```python
from build123d import *

# Parameters (mm, degrees)
F0_R          = 6.75
F0_R_2        = 2.15
F1_DEPTH      = 6
F1_DEPTH_BACK = 6
F3_START      = 5
F3_DEPTH      = 25
F4_SIZE2      = 3
F4_SIZE       = 1


with BuildPart() as f1:
    # F0 (on Top) → F1 (new body, two sides)
    with BuildSketch(Plane.XY) as f1_sk:
        Circle(F0_R)
        Circle(F0_R_2, mode=Mode.SUBTRACT)
    extrude(amount=F1_DEPTH)
    extrude(f1_sk.sketch, amount=-F1_DEPTH_BACK)

    # F2 (on Front) → F3 (join)
    with BuildSketch(Plane.XZ.offset(F3_START)):
        with BuildLine():
            ThreePointArc((1.5745130543, -4.2155555556), (3.6969790873, -2.5656082374), (4.5, 0))
            ThreePointArc((4.5, 0), (-2.5656082374, 3.6969790873), (-1.5745130543, -4.2155555556))
            ThreePointArc((-1.5745130543, -4.2155555556), (0, -2.9), (1.5745130543, -4.2155555556))
        make_face()
    extrude(amount=F3_DEPTH)

    # F4
    f4_edges = [f1.edges().sort_by_distance(p)[0] for p in [
        (0, -30, 4.5),
    ]]
    f4_side = f1.faces().sort_by_distance((0, -30, 0.234076))[0]
    chamfer(f4_edges, length=F4_SIZE, length2=F4_SIZE2, reference=f4_side)


solid = f1.part
```
Source: CAD feature listing. Evaluate the final solid. Frame: model axes, mm. A direction names the side the tool comes from. Give positions to 0.01 mm unless a question says otherwise; leave off trailing zeros. Loops run counter-clockwise (first coordinate to the right, second up) from the corner with the lowest first, then second, coordinate; pieces in that order, holes last. Notation, with made-up numbers: (-30.5, 65.25) - (-8.5, 65.25) arc R26 cw to (-8.5, 82.25) - close; hole circle Ø8 at (-21.5, -26). An arc over 180 degrees is marked (long way). Use CSV: the item, a comma, the result in double quotes. Start each with the question number.
1. Section C-C (y = -21.5). Output: boundary loops of the cut face in (x, z).
2. Reachability of faces 1 (the flat face through (-2, 2, -6)), 2 (the cylindrical face through (0, -18.1, -2.9)) from +Z, -Z, +X, -X, +Y, -Y: full face, straight path, thin tool, end or side. Return the list, or none.
3. Pin query (flat end, axial travel): pin 1 (3 mm diameter, centred on y = -6, z = 0, fed in from -X); pin 2 (1 mm diameter, centred on x = 1.5, y = -25.5, fed in from -Z); pin 3 (4 mm diameter, centred on x = 0, y = 0, fed in from +Z); pin 4 (2 mm diameter, centred on x = 3.5, z = -1.5, fed in from +Y). Return the tip coordinate at first contact, or that it passes through.
4. Ray query, L1, parallel to Y at x = 0, z = 3; L2, parallel to X at y = -1, z = -3.25; L3, parallel to X at y = -20, z = -4. Return the intervals inside material, ascending.
5. Draft query along X for faces 3 (the flat face through (-2, 2, 6)), 4 (the cylindrical face through (-2.15, 0.09, -0.08)). Return one class per face: +X half, -X half, draft (parallel to the pull), parting line (faces both ways), or undercut.
6. Section A-A (y = 0). Output: boundary loops of the cut face in (x, z), then the cut area to 3 significant figures.
7. Section B-B (x = 0). Output: boundary loops of the cut face in (y, z).
8. Section D-D (x = 5.75). Output: boundary loops of the cut face in (y, z), then the cut area to 3 significant figures.
Response:
1,outline,"(-1.57, -4.22) arc R1.6 cw to (1.57, -4.22) arc R4.5 ccw (long way) to start"
2,face 1,"-Z, +X, -X, +Y, -Y"
2,face 2,"-Z, -Y"
3,pin 1,"x = -5.03"
3,pin 2,"z = -4.22"
3,pin 3,"through"
3,pin 4,"y = 6.27"
4,L1,"-30 to -2.15, 2.15 to 6.75"
4,L2,"-6.68 to -1.9, 1.9 to 6.68"
4,L3,"-2.06 to -1.52, 1.52 to 2.06"
5,face 3,"draft"
5,face 4,"undercut"
6,outline,"(-6.75, -6) - (-2.15, -6) - (-2.15, 6) - (-6.75, 6) - close; (2.15, -6) - (6.75, -6) - (6.75, 6) - (2.15, 6) - close"
6,area,"110 mm²"
7,outline,"(-30, -2.9) - (-6.75, -2.9) - (-6.75, -6) - (-2.15, -6) - (-2.15, 6) - (-6.75, 6) - (-6.75, 4.5) - (-27, 4.5) - (-30, 3.5) - close; (2.15, -6) - (6.75, -6) - (6.75, 6) - (2.15, 6) - close"
8,outline,"(-3.54, -6) - (3.54, -6) - (3.54, 6) - (-3.54, 6) - close"
8,area,"84.9 mm²"
